Design review of the part built by this model. Coordinates are the model's own, in mm. A direction names the side the tool comes from. Give positions to 0.01 mm unless a question says otherwise; leave off trailing zeros. Loops run counter-clockwise (first coordinate to the right, second up) from the corner with the lowest first, then second, coordinate; pieces in that order, holes last. Notation, with made-up numbers: (75.25, -16.5) -> (94.25, -16.5) arc R16 ccw to (94.25, 14.5) -> close; hole circle Ø10 at (82, 48). An arc over 180 degrees is marked (long way). Answer as CSV lines item,"result".
from build123d import *

# Parameters (mm, degrees)
ESBO_O1_W                = 95
ESBO_O1_H                = 51
RESSALTO_EXTRUS_O1_DEPTH = 2
ESBO_O3_W                = 90
ESBO_O3_H                = 2
RESSALTO_EXTRUS_O3_DEPTH = 2
ESBO_O5_W                = 90
ESBO_O5_H                = 2
RESSALTO_EXTRUS_O4_DEPTH = 2
ESBO_O6_W                = 2
ESBO_O6_H                = 42
RESSALTO_EXTRUS_O5_DEPTH = 4
ESBO_O7_W                = 90
ESBO_O7_H                = 4
RESSALTO_EXTRUS_O6_DEPTH = 2
ESBO_O8_W                = 46
ESBO_O8_H                = 4
RESSALTO_EXTRUS_O7_DEPTH = 2.5
ESBO_O10_W               = 3.5
ESBO_O10_H               = 4
RESSALTO_EXTRUS_O8_DEPTH = 1.5
CORTE_EXTRUS_O1_DEPTH    = 52.5
CORTE_EXTRUS_O2_DEPTH    = 62.5


with BuildPart() as part:
    # Esboço1 → Ressalto-extrusão1 (new body)
    with BuildSketch(Plane(origin=(0, 0, 0), x_dir=(1, 0, 0), z_dir=(0, 1, 0))):
        with Locations((47.5, 25.5)):
            Rectangle(ESBO_O1_W, ESBO_O1_H)
    extrude(amount=RESSALTO_EXTRUS_O1_DEPTH)

    # Esboço3 → Ressalto-extrusão3 (add)
    with BuildSketch(Plane(origin=(0, 0, 0), x_dir=(-1, 0, 0), z_dir=(0, -1, 0))):
        with Locations((-47.5, 5.5)):
            Rectangle(ESBO_O3_W, ESBO_O3_H)
    extrude(amount=RESSALTO_EXTRUS_O3_DEPTH)

    # Esboço5 → Ressalto-extrusão4 (add)
    with BuildSketch(Plane.XZ):
        with Locations((47.5, -45.5)):
            Rectangle(ESBO_O5_W, ESBO_O5_H)
    extrude(amount=RESSALTO_EXTRUS_O4_DEPTH)

    # Esboço6 → Ressalto-extrusão5 (add)
    with BuildSketch(Plane.XZ):
        with Locations((91.5, -25.5)):
            Rectangle(ESBO_O6_W, ESBO_O6_H)
    extrude(amount=RESSALTO_EXTRUS_O5_DEPTH)

    # Esboço7 → Ressalto-extrusão6 (add)
    with BuildSketch(Plane(origin=(0, -2, 0), x_dir=(-1, 0, 0), z_dir=(0, -1, 0))):
        with Locations((-47.5, 4.5)):
            Rectangle(ESBO_O7_W, ESBO_O7_H)
        with Locations((-47.5, 46.5)):
            Rectangle(ESBO_O7_W, ESBO_O7_H)
    extrude(amount=RESSALTO_EXTRUS_O6_DEPTH)

    # Esboço8 → Ressalto-extrusão7 (add)
    with BuildSketch(Plane.ZY):
        with Locations((-25.5, -2)):
            Rectangle(ESBO_O8_W, ESBO_O8_H)
    extrude(amount=-RESSALTO_EXTRUS_O7_DEPTH)

    # Esboço10 → Ressalto-extrusão8 (add)
    with BuildSketch(Plane.XZ.offset(4)):
        with Locations((4.25, -4.5)):
            Rectangle(ESBO_O10_W, ESBO_O10_H)
        with Locations((4.25, -46.5)):
            Rectangle(ESBO_O10_W, ESBO_O10_H)
    extrude(amount=RESSALTO_EXTRUS_O8_DEPTH)

    # Esboço12 → Corte-extrusão1 (cut)
    with BuildSketch(Plane.XY.offset(-2.5)):
        Polygon((2.5, -4), (4.25, -5.5), (2.5, -5.5), align=None)
    extrude(amount=-CORTE_EXTRUS_O1_DEPTH, mode=Mode.SUBTRACT)

    # Esboço13 → Corte-extrusão2 (cut)
    with BuildSketch(Plane.XY.offset(-2.5)):
        Polygon((4.25, -5.5), (6, -4), (6, -5.5), align=None)
    extrude(amount=-CORTE_EXTRUS_O2_DEPTH, mode=Mode.SUBTRACT)


solid = part.part
Q1. To check wall thickness, follow probe 1 along X at (y, z) = (-3.5, -43); probe 2 along Z at (x, y) = (42.5, -1); probe 3 along Y at (x, z) = (61.5, -3). State the ranges of each line that lie inside material, in increasing order. Write a range as from..to.
Filled sheet:
probe 1,"x = 0..2.5, 90.5..92.5"
probe 2,"z = -46.5..-44.5, -6.5..-4.5"
probe 3,"y = -4..-2, 0..2"
Q2. Clearance check with flat-ended pins moving along their axes: pin 1 Ø4 at (y, z) = (-2.5, -18.5) entering from +X; pin 2 Ø1.5 at (x, z) = (48.5, -21) entering from -Y; pin 3 Ø23 at (x, z) = (65.5, -34) entering from -Y. State where each tip first meets the part, or that it passes through.
Filled sheet:
pin 1,"stops at x = 92.5"
pin 2,"stops at y = 0"
pin 3,"stops at y = -4"
Q3. For faces 4 (the flat face through (92.5, -2, -25)), 5 (the flat face through (46, 0, -26)), 6 (the flat face through (46, -3, -2.5)), list the 3-axis set-ups (+Z, -Z, +X, -X, +Y, -Y) from which the entire face can be reached by the end or side of a thin tool; tool diameter is ignored.
Filled sheet:
face 4,"+Z, -Z, +X, -Y"
face 5,"-Y"
face 6,"+Z, +X, -X, -Y"
Q4. We need section A-A, the plane x = 14. State the section outline as (y, z) points.
Filled sheet:
outline,"(-4, -48.5) -> (-2, -48.5) -> (-2, -46.5) -> (0, -46.5) -> (0, -51) -> (2, -51) -> (2, 0) -> (0, 0) -> (0, -4.5) -> (-2, -4.5) -> (-2, -2.5) -> (-4, -2.5) -> (-4, -6.5) -> (0, -6.5) -> (0, -44.5) -> (-4, -44.5) -> close"
Q5. We need section B-B, the plane z = -18. State the section outline as (x, y) points, and give its area (3 significant figures).
Filled sheet:
outline,"(0, -4) -> (2.5, -4) -> (2.5, 0) -> (90.5, 0) -> (90.5, -4) -> (92.5, -4) -> (92.5, 0) -> (95, 0) -> (95, 2) -> (0, 2) -> close"
area,"208 mm^2"
Q6. The part is to be moulded in two halves that separate along Y. For faces 1 (the flat face through (47, 2, -26)), 2 (the flat face through (47, -1, -4.5)), 3 (the flat face through (5.113, -4.76, -4.472)), say which applies: pulls with the +Y half, pulls with the -Y half, needs draft (parallel to the pull), parting line crosses it, or undercut.
Filled sheet:
face 1,"pulls with the +Y half"
face 2,"undercut"
face 3,"pulls with the -Y half"
